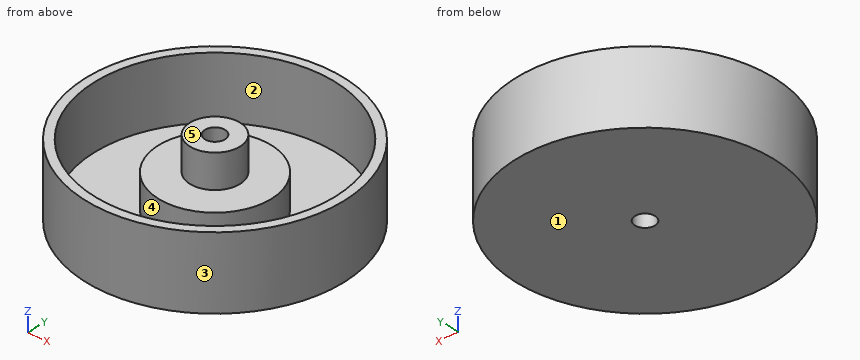
Autodesk Fusion 360 part; units mm, degrees
sketch "Sketch1" plane through (0, 0, 0) normal (0, 0, 1) x (1, 0, 0)
  circle A0 centre (0, 0) radius 15.45
  circle A1 centre (0, 0) radius 14.4
  circle A2 centre (0, 0) radius 6.75
  circle A3 centre (0, 0) radius 3
  circle A4 centre (0, 0) radius 1.2
  dimension "d24" = 30.9
  dimension "d25" = 28.8
  dimension "d26" = 13.5
  dimension "d27" = 6
  dimension "d28" = 2.4
extrude "Extrude1" add sketch "Sketch1" along normal blind 1.2 contours A1 makes body 1
extrude "Extrude2" add sketch "Sketch1" along normal blind 8.7 contours A0 bodies 1
extrude "Extrude3" add sketch "Sketch1" along normal blind 9.2 separate body contours A3 makes body 2
extrude "Extrude4" add sketch "Sketch1" along normal blind 5.2 contours A2 bodies 1 2
equation "d25 = 30.9 mm - 2.1 mm"
equation "d35 = 9.2 mm - 4 mm"
Here's how the part is built. I have some questions about the finished solid (model axes, mm). Face numbers are marked on the shaded views. A direction names the side the tool comes from. Round coordinates to 2 decimals unless told otherwise and drop trailing zeros. Write each loop counter-clockwise with the first axis right and the second up, starting at its lowest first coordinate (ties: lowest second). Pieces come first, ordered by that corner, then holes.
1. I need wall thicknesses on L1, parallel to Y at x = 0, z = 4.5; L2, parallel to Y at x = 5, z = 2.5; L3, parallel to Y at x = -6, z = 2.5. Which ranges of each line are inside material? Lowest first, please.
2. For the marked faces 1 and 2, which set-ups out of +Z, -Z, +X, -X, +Y, -Y let a thin tool reach every point of the face, with its end or its side?
3. Suppose I cut it at A-A (y = 0). List the corners of the cut face in (x, z) for me.
4. Suppose I cut it at D-D (x = -10). List the corners of the cut face in (y, z) for me.
5. Will these pins go through, and if not, where does the flat tip stop? pin 1 Ø2 at (y, z) = (-8, 6) entering from -X; pin 2 Ø4 at (x, z) = (9.5, 1) entering from +Y; pin 3 Ø5 at (x, z) = (12, 4) entering from +Y.
6. If we mould it in two halves opening along Y, with no side actions, what happens to the marked faces 3, 4 and 5? For each: released by +Y, released by -Y, zero draft, split by the parting line, or undercut.
7. Suppose I cut it at C-C (z = 6). List the corners of the cut face in (x, y) for me, and give its area (3 significant figures).
Answer sheet:
1. L1: y = -15.45 to -14.4, -6.75 to -1.2, 1.2 to 6.75, 14.4 to 15.45
1. L2: y = -14.62 to -13.5, -4.53 to 4.53, 13.5 to 14.62
1. L3: y = -14.24 to -13.09, -3.09 to 3.09, 13.09 to 14.24
2. face 1: -Z, +X, -X, +Y, -Y
2. face 2: +Z
3. outline: (-15.45, 0) - (-1.2, 0) - (-1.2, 9.2) - (-3, 9.2) - (-3, 5.2) - (-6.75, 5.2) - (-6.75, 1.2) - (-14.4, 1.2) - (-14.4, 8.7) - (-15.45, 8.7) - close; (1.2, 0) - (15.45, 0) - (15.45, 8.7) - (14.4, 8.7) - (14.4, 1.2) - (6.75, 1.2) - (6.75, 5.2) - (3, 5.2) - (3, 9.2) - (1.2, 9.2) - close
4. outline: (-11.78, 0) - (11.78, 0) - (11.78, 8.7) - (10.36, 8.7) - (10.36, 1.2) - (-10.36, 1.2) - (-10.36, 8.7) - (-11.78, 8.7) - close
5. pin 1: stops at x = -13.77
5. pin 2: stops at y = 13.51
5. pin 3: stops at y = 12.18
6. face 3: split by the parting line
6. face 4: undercut
6. face 5: zero draft
7. outline: circle Ø30.9 at (0, 0); circle Ø6 at (0, 0); hole circle Ø28.8 at (0, 0); hole circle Ø2.4 at (0, 0)
7. area: 122 mm2
